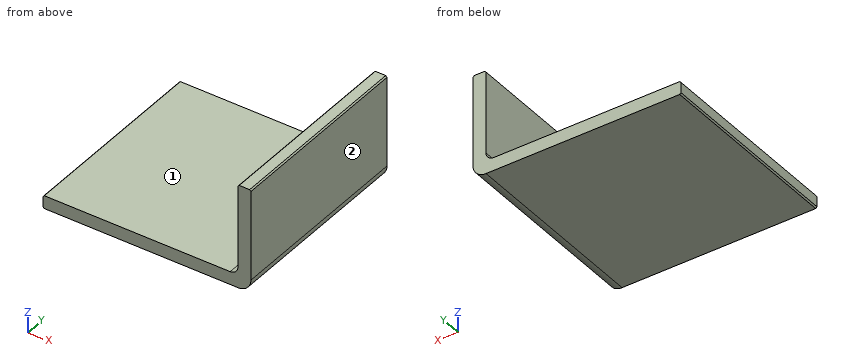
```python
from build123d import *

# Parameters (mm, degrees)
F1_DEPTH = 381
F2_SIZE  = 2.54


with BuildPart() as f1:
    # F0 (on Front) → F1 (new body)
    with BuildSketch(Plane.XZ):
        with BuildLine():
            Line((388.178844, 25.4), (22.418844, 25.4))
            Line((22.418844, 25.4), (22.418844, 0))
            Line((22.418844, 0), (403.418844, 0))
            ThreePointArc((403.418844, 0), (421.379356, 7.439488), (428.818844, 25.4))
            Line((428.818844, 25.4), (428.818844, 203.2))
            Line((428.818844, 203.2), (403.418844, 203.2))
            Line((403.418844, 203.2), (403.418844, 40.64))
            ThreePointArc((403.418844, 40.64), (398.955151, 29.863693), (388.178844, 25.4))
        make_face()
    extrude(amount=F1_DEPTH)

    # F2
    f2_edges = [f1.edges().sort_by_distance(p)[0] for p in [
        (22.418844, -190.5, 0),
        (22.418844, -190.5, 25.4),
        (428.818844, -190.5, 203.2),
        (403.418844, -190.5, 203.2),
    ]]
    chamfer(f2_edges, length=F2_SIZE)


solid = f1.part
```
Design review of the part built by this model. Coordinates are the model's own, in mm. Face numbers are marked on the shaded views. A direction names the side the tool comes from. Coordinates: 2 decimals unless noted, no trailing zeros. Loops run counter-clockwise (first coordinate to the right, second up) from the corner with the lowest first, then second, coordinate; pieces in that order, holes last.
Q1. We need section B-B on x = 362. State the section outline as (y, z) points.
Reported:
outline: (-381, 0) - (0, 0) - (0, 25.4) - (-381, 25.4) - close
Q2. To check wall thickness, follow line 1 (Z direction, x = 224, y = -357.5); line 2 (X direction, y = -337.5, z = 159); line 3 (Z direction, x = 399, y = -98.5). State the ranges of each line that lie inside material, in increasing order.
Reported:
line 1: z = 0 to 25.4
line 2: x = 403.42 to 428.82
line 3: z = 0 to 29.91
Q3. We need section C-C on z = 175. State the section outline as (x, y) points.
Reported:
outline: (403.42, -381) - (428.82, -381) - (428.82, 0) - (403.42, 0) - close
Q4. We need section A-A on y = -156. State the section outline as (x, z) points, and give its area (3 significant figures).
Reported:
outline: (22.42, 2.54) - (24.96, 0) - (403.42, 0) arc R25.4 ccw to (428.82, 25.4) - (428.82, 200.66) - (426.28, 203.2) - (405.96, 203.2) - (403.42, 200.66) - (403.42, 40.64) arc R15.24 cw to (388.18, 25.4) - (24.96, 25.4) - (22.42, 22.86) - close
area: 14,700 mm2
Q5. Tool access review of the marked faces 1 and 2: name each direction out of +Z, -Z, +X, -X, +Y, -Y from which nothing blocks a thin tool from reaching the whole face with its end or side.
Reported:
face 1: +Z, -X, +Y, -Y
face 2: +Z, -Z, +X, +Y, -Y
Q6. For pin 1 (10 mm diameter, centred on y = -51.5, z = 52, fed in from -X); pin 2 (8 mm diameter, centred on x = 246, y = -201, fed in from +Z), all flat-tipped, find the tip position at first contact; note any pin that passes through.
Reported:
pin 1: stops at x = 403.42
pin 2: stops at z = 25.4
